For this review, take the finished solid that the model builds, in its own axes (mm). Round coordinates to 2 decimals unless told otherwise and drop trailing zeros. Write each loop counter-clockwise with the first axis right and the second up, starting at its lowest first coordinate (ties: lowest second). Pieces come first, ordered by that corner, then holes. Notation, with made-up numbers: (37, 67) -> (79, 67) arc R29 ccw to (79, 105) -> close; hole circle Ø7 at (-17, -10.75). An arc over 180 degrees is marked (long way). Answer in a Markdown table with one row per item. Add a question column.
Autodesk Inventor part; units mm, degrees
ref_plane "YZ Plane" through (0, 0, 0) normal (1, 0, 0) x (0, 1, 0)
ref_plane "XZ Plane" through (0, 0, 0) normal (0, 1, 0) x (-1, 0, 0)
ref_plane "XY Plane" through (0, 0, 0) normal (0, 0, 1) x (1, 0, 0)
sketch "Эскиз1" plane through (0, 0, 0) normal (0, 0, 1) x (1, 0, 0)
  line L0 (0, 0) -> (10, 0)
  line L1 (10, 0) -> (10, 3)
  line L2 (10, 3) -> (0, 3)
  line L3 (0, 3) -> (0, 0)
  dimension "d0" = 10
  dimension "d1" = 3
extrude "Выдавливание1" add sketch "Эскиз1" along normal blind 3
pattern_linear "Прямоуг.массив1" count 11 spacing 20 along (1, 0, 0) of "Выдавливание1"
sketch "Эскиз2" plane through (0, 0, 3) normal (0, 0, 1) x (1, 0, 0)
  line L0 (0, 3) -> (0, 0)
  line L1 (0, 3) -> (220, 3)
  line L2 (220, 3) -> (220, 73)
  line L3 (220, 73) -> (0, 73)
  line L4 (0, 73) -> (0, 3)
  line L5 (210, 0) -> (210, 3)
  dimension "d8" = 70
  dimension "d11" = 10
extrude "Выдавливание2" add sketch "Эскиз2" against normal blind 3
sketch "Эскиз3" plane through (0, 0, 3) normal (0, 0, 1) x (1, 0, 0)
  line L0 (0, 73) -> (220, 73)
  line L1 (220, 73) -> (217, 73)
  line L2 (217, 73) -> (217, 63)
  line L3 (217, 63) -> (220, 63)
  line L4 (220, 63) -> (220, 73)
  point P0 (0, 0)
  dimension "d12" = 3
  dimension "d13" = 10
extrude "Выдавливание3" cut sketch "Эскиз3" against normal blind 10
pattern_linear "Прямоуг.массив2" count 4 spacing 20 along (0, -1, 0) of "Выдавливание3"
sketch "Эскиз4" plane through (0, 0, 3) normal (0, 0, 1) x (1, 0, 0)
  line L0 (0, 73) -> (217, 73)
  line L1 (0, 73) -> (10, 73)
  line L2 (10, 73) -> (10, 70)
  line L3 (10, 70) -> (0, 70)
  line L4 (0, 70) -> (0, 73)
  point P0 (0, 0)
  dimension "d19" = 10
  dimension "d20" = 3
extrude "Выдавливание4" cut sketch "Эскиз4" against normal blind 10
pattern_linear "Прямоуг.массив3" count 11 spacing 20 along (1, 0, 0) of "Выдавливание4"
properties part number "000.102 - Left wall"
1. We need section A-A (x = 117.5). Write out the cut boundary in (y, z), plus the area to 3 significant figures.
2. Clearance check with flat-ended pins moving along their axes: pin 1 Ø0.9 at (x, z) = (143.5, 1.5) entering from +Y; pin 2 Ø1.5 at (y, z) = (52, 2) entering from -X; pin 3 Ø0.9 at (y, z) = (71.5, 1.5) entering from -X; pin 4 Ø1.5 at (x, z) = (91, 2.5) entering from -Y. State where each tip first meets the part, or that it passes through.
3. For L1, parallel to Y at x = 131, z = 0.9; L2, parallel to Y at x = 200.5, z = 2.1; L3, parallel to X at y = 47, z = 2.6, list the stretches that pass through material, from the lowest coordinate up. Write a range as [from, to].
Response:
| question | item | result |
|---|---|---|
| 1 | outline | (3, 0) -> (73, 0) -> (73, 3) -> (3, 3) -> close |
| 1 | area | 210 mm2 |
| 2 | pin 1 | y = 70 |
| 2 | pin 2 | x = 0 |
| 2 | pin 3 | x = 10 |
| 2 | pin 4 | y = 3 |
| 3 | L1 | [3, 73] |
| 3 | L2 | [0, 70] |
| 3 | L3 | [0, 217] |
